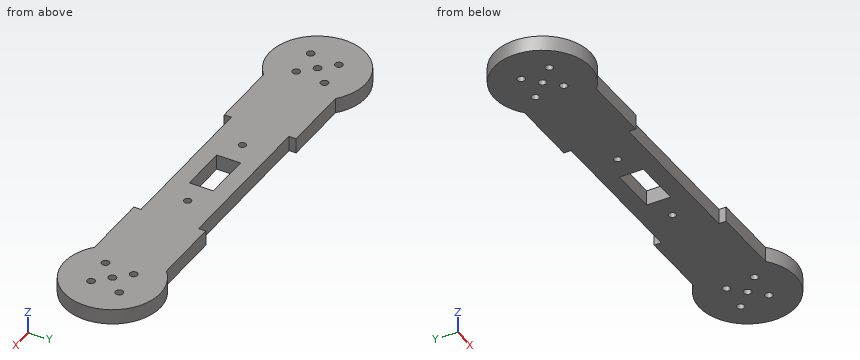
```python
from build123d import *

# Parameters (mm, degrees)
SKETCH3_R                = 1.5
SKETCH3_W                = 20
SKETCH3_H                = 10
BOSS_EXTRUDE1_DEPTH      = 6.35
M3_CLEARANCE_HOLE1_D     = 3.2
M3_CLEARANCE_HOLE1_DEPTH = 7.5
M3_CLEARANCE_HOLE1_TIP   = 0.96137699
SKETCH4_W                = 66
SKETCH4_H                = 3
CUT_EXTRUDE1_DEPTH       = 10


with BuildPart() as part:
    # Sketch3 → Boss-Extrude1 (new body)
    with BuildSketch(Plane.XY):
        with BuildLine():
            Line((61.771243445, -15), (-61.771243445, -15))
            ThreePointArc((-61.771243445, -15), (-95, 0), (-61.771243445, 15))
            Line((-61.771243445, 15), (61.771243445, 15))
            ThreePointArc((61.771243445, 15), (95, 0), (61.771243445, -15))
        make_face()
        with Locations((-20, 0)):
            Circle(SKETCH3_R, mode=Mode.SUBTRACT)
        with Locations((20, 0)):
            Circle(SKETCH3_R, mode=Mode.SUBTRACT)
        Rectangle(SKETCH3_W, SKETCH3_H, mode=Mode.SUBTRACT)
    extrude(amount=BOSS_EXTRUDE1_DEPTH)

    # M3 Clearance Hole1
    with Locations(Plane(origin=(0, 0, 0), x_dir=(-1, 0, 0), z_dir=(0, 0, -1))):
        with Locations((81.717514421, -6.717514421), (75, 0), (0, 0), (-75, 0), (-69.343145751, 5.656854249), (-80.656854249, -5.656854249), (-81.717514421, 6.717514421), (-68.282485579, -6.717514421), (68.282485579, 6.717514421), (80.656854249, 5.656854249), (69.343145751, -5.656854249)):
            Hole(M3_CLEARANCE_HOLE1_D / 2, depth=M3_CLEARANCE_HOLE1_DEPTH)
            with Locations((0, 0, -(M3_CLEARANCE_HOLE1_DEPTH + M3_CLEARANCE_HOLE1_TIP / 2))):  # 118° drill point
                Cone(0, M3_CLEARANCE_HOLE1_D / 2, M3_CLEARANCE_HOLE1_TIP, mode=Mode.SUBTRACT)

    # Sketch4 → Cut-Extrude1 (cut)
    with BuildSketch(Plane(origin=(0, 0, 0), x_dir=(-1, 0, 0), z_dir=(0, 0, -1))):
        with Locations((0, 13.5)):
            Rectangle(SKETCH4_W, SKETCH4_H)
    cut_extrude1 = extrude(amount=-CUT_EXTRUDE1_DEPTH, mode=Mode.SUBTRACT)

    # Mirror1: Cut-Extrude1 across plane
    add(cut_extrude1.mirror(Plane.ZX), mode=Mode.SUBTRACT)


solid = part.part
```
Geometry check sheet. Reference: the model listing, model coordinates, mm. Round coordinates to 2 decimals unless told otherwise and drop trailing zeros. Order: outer loops, then holes, each group sorted by start corner. A loop starts at its lowest first (then second) coordinate and runs counter-clockwise, first axis right, second up. Notation, with made-up numbers: (-18.5, -28.75) - (14.5, -28.75) arc R23 ccw to (14.5, 2.25) - close; hole circle Ø3 at (-38, 17.5). An arc over 180 degrees is marked (long way). Use a Markdown table: item, result. Add a question column.
(1) Sectioned sample at B-B, the plane z = 1.5. Count the separate pieces of the cut face and the enclosed holes in it, and give its area (3 significant figures).
(2) Depth check by flat-ended pin: pin 1 (12 mm diameter, centred on x = 68.5, y = 3, fed in from -Z); pin 2 (0.9 mm diameter, centred on y = 13, z = 2.5, fed in from +X); pin 3 (1.9 mm diameter, centred on x = -41, z = 3, fed in from -Y); pin 4 (1.9 mm diameter, centred on x = -9.5, z = 3, fed in from +Y). Enter the tip coordinate at first touch or a pass-through.
(3) Material ranges on line 1 along Y through (x, z) = (82, 0.5) (3 decimals); line 2 along Y through (x, z) = (17.5, 5.5); line 3 along X through (y, z) = (17, 2), recorded low to high. Write a range as [from, to].
(4) Sectioned sample at A-A, the plane x = 75. Enter the section's corners in (y, z), and give its area (3 significant figures).
(5) Sectioned sample at C-C, the plane x = 43. Enter the section's corners in (y, z), and give its area (4 significant figures).
Answers below:
| question | item | result |
|---|---|---|
| 1 | separate pieces | 1 |
| 1 | enclosed holes | 13 |
| 1 | area | 5,250 mm² |
| 2 | pin 1 | z = 0 |
| 2 | pin 2 | x = 90.57 |
| 2 | pin 3 | y = -15 |
| 2 | pin 4 | y = 12 |
| 3 | line 1 | [-18.735, -6.526], [-4.787, 5.143], [8.292, 18.735] |
| 3 | line 2 | [-12, 12] |
| 3 | line 3 | [-85.54, -64.46], [64.46, 85.54] |
| 4 | outline | (-20, 0) - (-1.6, 0) - (-1.6, 6.35) - (-20, 6.35) - close; (1.6, 0) - (20, 0) - (20, 6.35) - (1.6, 6.35) - close |
| 4 | area | 234 mm² |
| 5 | outline | (-15, 0) - (15, 0) - (15, 6.35) - (-15, 6.35) - close |
| 5 | area | 190.5 mm² |
